from build123d import *

# Parameters (mm, degrees)
BOSS_EXTRUDE1_DEPTH = 38.1
FILLET1_R           = 19.05
SKETCH2_R           = 2.667
CUT_EXTRUDE1_DEPTH  = 54.127911685
FILLET2_R           = 6.35
SKETCH3_R           = 2.667
CUT_EXTRUDE2_DEPTH  = 55.34724579
FILLET3_R           = 3.175
CHAMFER1_SIZE       = 1.5875
CHAMFER2_SIZE       = 0.79375


with BuildPart() as part:
    # Sketch1 → Boss-Extrude1 (new body)
    with BuildSketch(Plane.XY):
        Polygon((-3.175, 31.75), (3.175, 31.75), (3.175, 6.35), (19.05, 6.35), (19.05, 0), (-19.05, 0), (-19.05, 6.35), (-3.175, 6.35), align=None)
    extrude(amount=BOSS_EXTRUDE1_DEPTH)

    # Fillet1
    fillet1_edges = [part.edges().sort_by_distance(p)[0] for p in [
        (0, 31.75, 0),
        (0, 31.75, 38.1),
    ]]
    fillet(fillet1_edges, radius=FILLET1_R - 0.0001)  # a hair under: the kernel refuses the full size

    # Sketch2 → Cut-Extrude1 (cut, through all)
    with BuildSketch(Plane.XZ):
        with Locations((12.7, 31.75)):
            Circle(SKETCH2_R)
        with Locations((12.7, 6.35)):
            Circle(SKETCH2_R)
        with Locations((-12.7, 6.35)):
            Circle(SKETCH2_R)
        with Locations((-12.7, 31.75)):
            Circle(SKETCH2_R)
    extrude(amount=-CUT_EXTRUDE1_DEPTH, mode=Mode.SUBTRACT)

    # Fillet2
    fillet2_edges = [part.edges().sort_by_distance(p)[0] for p in [
        (19.05, 3.175, 0),
        (-19.05, 3.175, 0),
        (19.05, 3.175, 38.1),
        (-19.05, 3.175, 38.1),
    ]]
    fillet(fillet2_edges, radius=FILLET2_R)

    # Sketch3 → Cut-Extrude2 (cut, through all)
    with BuildSketch(Plane.ZY.offset(3.175)):
        with Locations(Location((19.05, 22.225, 0), (0, 0, 270))):
            Circle(SKETCH3_R)
    extrude(amount=-CUT_EXTRUDE2_DEPTH, mode=Mode.SUBTRACT)

    # Fillet3
    fillet3_edges = [part.edges().sort_by_distance(p)[0] for p in [
        (-3.175, 6.35, 19.05),
        (3.175, 6.35, 19.05),
    ]]
    fillet(fillet3_edges, radius=FILLET3_R)

    # Chamfer1
    chamfer1_edges = [part.edges().sort_by_distance(p)[0] for p in [
        (-3.175, 11.11255, 0),
        (-3.175, 11.11255, 38.1),
        (-3.175, 26.170413471, 32.520413471),
        (-3.175, 26.170413471, 5.579586529),
        (3.175, 26.170413471, 32.520413471),
        (3.175, 26.170413471, 5.579586529),
        (-19.05, 6.35, 19.05),
        (9.525, 6.35, 0),
        (-17.190128061, 6.35, 36.240128061),
        (-17.190128061, 6.35, 1.859871939),
        (19.05, 6.35, 19.05),
        (9.525, 6.35, 38.1),
        (17.190128061, 6.35, 36.240128061),
        (17.190128061, 6.35, 1.859871939),
        (3.175, 11.11255, 0),
        (3.175, 11.11255, 38.1),
        (-9.525, 6.35, 0),
        (-9.525, 6.35, 38.1),
        (4.10493597, 7.27993597, 0),
        (4.10493597, 7.27993597, 38.1),
        (-4.10493597, 7.27993597, 0),
        (-4.10493597, 7.27993597, 38.1),
    ]]
    chamfer(chamfer1_edges, length=CHAMFER1_SIZE)

    # Chamfer2
    chamfer2_edges = [part.edges().sort_by_distance(p)[0] for p in [
        (-15.367, 6.35, 31.75),
        (-15.367, 6.35, 6.35),
        (10.033, 6.35, 6.35),
        (10.033, 6.35, 31.75),
        (3.175, 24.892, 19.05),
        (-3.175, 24.892, 19.05),
    ]]
    chamfer(chamfer2_edges, length=CHAMFER2_SIZE)


solid = part.part
Here's how the part is built. I have some questions about the finished solid (model axes, mm). A direction names the side the tool comes from. Round coordinates to 2 decimals unless told otherwise and drop trailing zeros. One line per item, written item: value.
1) I'm going to push flat-ended pins straight in: pin 1 Ø12 at (y, z) = (11.5, 13.5) entering from +X; pin 2 Ø2 at (x, y) = (-3, 17.5) entering from +Z; pin 3 Ø6 at (y, z) = (16.5, 18.5) entering from -X (3 decimals). Where does each tip first touch, or does it pass through?
Filled sheet:
pin 1: stops at x = 18.31
pin 2: stops at z = 37.09
pin 3: stops at x = -3.175
2) We'd pull the mould along Z, two halves only. Please class faces 3 (the face through (4.13, 7.255, 19.294)), 4 (the face through (-3.65, 6.88, 37.12)), 5 (the face through (2.37, 11.09, 0.78)), 6 (the face through (12.4, 2.7, 34.4)): released by +Z, released by -Z, zero draft, split by the parting line, or undercut.
Filled sheet:
face 3: zero draft
face 4: released by +Z
face 5: released by -Z
face 6: undercut
3) Suppose I cut it at A-A on x = -11. Give the number of separate pieces and of enclosed holes in the cut face, plus the area to 3 significant figures.
Filled sheet:
separate pieces: 3
enclosed holes: 0
area: 186 mm2
4) For faces 1 (the face through (17.14, 2.35, 1.81)), 2 (the face through (-9.569, 5.567, 0.805)), which set-ups out of +Z, -Z, +X, -X, +Y, -Y let a thin tool reach every point of the face, with its end or its side?
Filled sheet:
face 1: -Z, +X, +Y, -Y
face 2: -Z, -X, +Y
5) If I drill on line 1 (Z direction, x = -12.7, y = 2.6); line 2 (X direction, y = 2.5, z = 6); line 3 (Y direction, x = -16.5, z = 8.5), over which ranges is the centre line in solid material (lowest first)? Write a range as [from, to].
Filled sheet:
line 1: z = [0, 3.68], [9.02, 29.08], [34.42, 38.1]
line 2: x = [-19.04, -15.34], [-10.06, 10.06], [15.34, 19.04]
line 3: y = [0, 6.35]
